The listing builds one solid part. Answer for the finished solid, in the listing's coordinates (mm). Face numbers are marked on the shaded views. A direction names the side the tool comes from. Round coordinates to 2 decimals unless told otherwise and drop trailing zeros. Loops run counter-clockwise (first coordinate to the right, second up) from the corner with the lowest first, then second, coordinate; pieces in that order, holes last. Notation, with made-up numbers: M 16,53.5 L 73,53.5 A8 cw 73,62.5 Z; hole C 48.25,17.5 d11. An arc over 180 degrees is marked long. Answer as a JSON object with one key per item and string values.
```python
from build123d import *

# Parameters (mm, degrees)
CHAMFER_1_SIZE = 0.5


with BuildPart() as part:
    # 草图1 → 旋转1 (revolve)
    with BuildSketch(Plane.XY):
        Polygon((-12.301369863, 0.334637965), (-12.301369863, 8.334637965), (-10.301369863, 8.334637965), (-10.301369863, 4.334637965), (24.698630137, 4.334637965), (24.698630137, 3.334637965), (27.698630137, 3.334637965), (27.698630137, 0.334637965), align=None)
    revolve(axis=Axis((27.698630137, 0.334637965, 0), (-1, 0, 0)))

    # 倒角1
    chamfer_1_edges = [part.edges().sort_by_distance(p)[0] for p in [
        (27.698630137, -2.665362035, 0),
        (-12.301369863, -7.665362035, 0),
    ]]
    chamfer(chamfer_1_edges, length=CHAMFER_1_SIZE)


solid = part.part
```
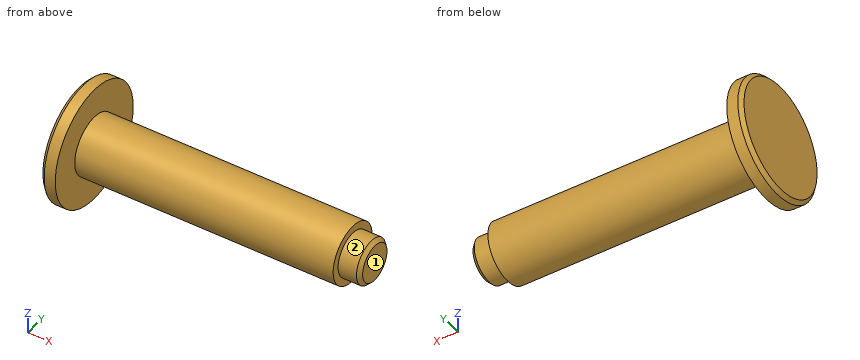
Item 1: Which of the six approach directions +Z, -Z, +X, -X, +Y, -Y give full straight-line access (tool end or side, diameter ignored) to the marked faces 1 and 2?
Values follow:
{"face 1": "+Z, -Z, +X, +Y, -Y", "face 2": "+X"}
Item 2: The part is cut by section B-B (x = 0). Give the vertices of the cut face in (y, z), then the cut area to 3 significant figures.
Values follow:
{"outline": "C 0.33,0 d8", "area": "50.3 mm^2"}
Item 3: Flat-ended cylindrical pins translate along their axes: P1, Ø1.5, axis at x = 7.5, y = -3.5, coming from the -Z side; P2, Ø4, axis at x = -4.5, z = 3, coming from the +Y side; P3, Ø8, axis at x = 15.5, y = -3, coming from the -Z side; P4, Ø4, axis at y = 2.5, z = 2, coming from the +X side. Find the tip coordinate at first contact, or state that the pin passes through.
Values follow:
{"P1": "z = -2.55", "P2": "y = 4.21", "P3": "z = -4", "P4": "x = 27.7"}
Item 4: The part is cut by section A-A (z = 0). Give the vertices of the cut face in (x, y), then the cut area to 4 significant figures.
Values follow:
{"outline": "M -12.3,-7.17 L -11.8,-7.67 L -10.3,-7.67 L -10.3,-3.67 L 24.7,-3.67 L 24.7,-2.67 L 27.2,-2.67 L 27.7,-2.17 L 27.7,2.83 L 27.2,3.33 L 24.7,3.33 L 24.7,4.33 L -10.3,4.33 L -10.3,8.33 L -11.8,8.33 L -12.3,7.83 Z", "area": "329.5 mm^2"}
Item 5: Straight lines are drawn through the part: line 1 (X direction, y = 1, z = 5.75); line 2 (Y direction, x = 11, z = 0); line 3 (Z direction, x = 7, y = 0.5). For each, find the intervals that lie inside material, in ascending order.
Values follow:
{"line 1": "-12.3 to -10.3", "line 2": "-3.67 to 4.33", "line 3": "-4 to 4"}
